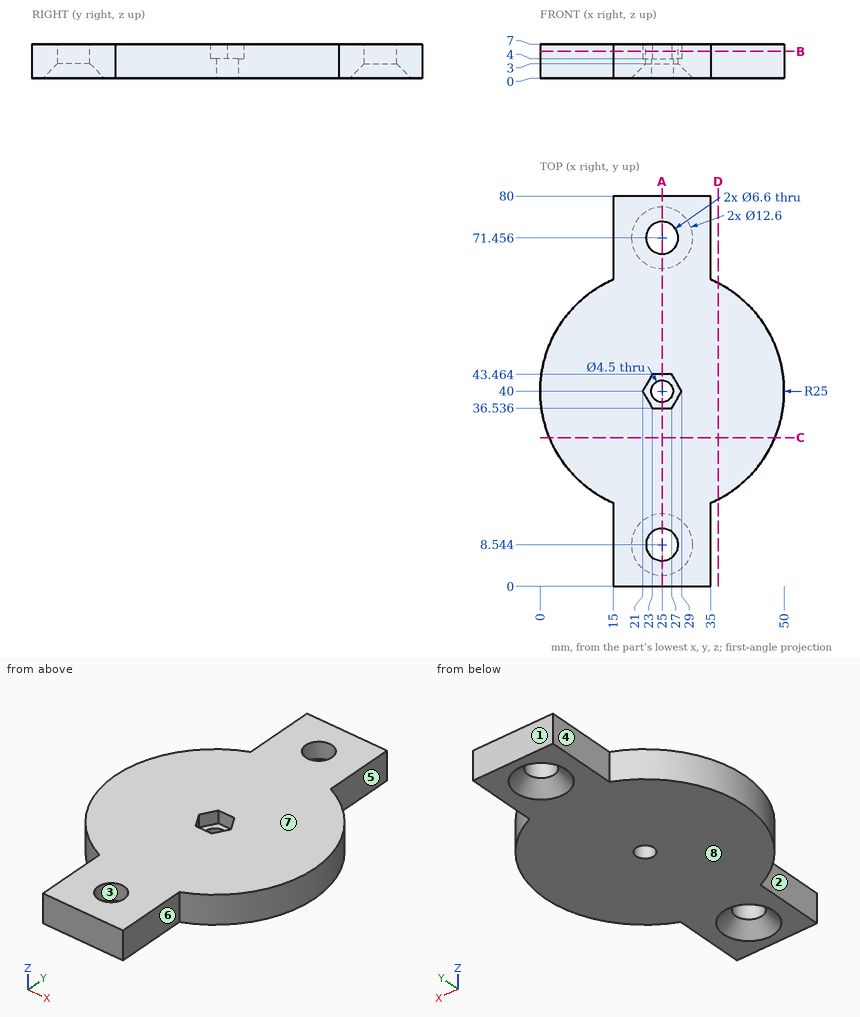
Study the drawing (mm; zero at the part's minimum x, y, z) and answer. A direction names the side the tool comes from. Give positions to 0.01 mm unless a question says otherwise; leave off trailing zeros. Order: outer loops, then holes, each group sorted by start corner. A loop starts at its lowest first (then second) coordinate and runs counter-clockwise, first axis right, second up.
1. The mould has two halves that part along Z. Classify the marked faces 6, 7 and 8: released by +Z, released by -Z, zero draft, split by the parting line, or undercut.
Result sheet:
face 6: zero draft
face 7: released by +Z
face 8: released by -Z
2. For the marked faces 1, 2, 3, 4 and 5, determine the directions among +Z, -Z, +X, -X, +Y, -Y from which every point of the face is accessible in a straight line to the end or side of a thin tool.
Result sheet:
face 1: +Z, -Z, +X, -X, +Y
face 2: +Z, -Z, -X, -Y
face 3: +Z, -Z
face 4: +Z, -Z, -X, +Y
face 5: +Z, -Z, +X, +Y
3. Section A-A, the plane x = 25 is taken. Determine the outline of the cut face in (y, z), and give its area (3 significant figures).
Result sheet:
outline: (0, 0) - (2.24, 0) - (5.24, 3) - (5.24, 7) - (0, 7) - close; (11.84, 3) - (14.84, 0) - (37.75, 0) - (37.75, 4) - (36.54, 4) - (36.54, 7) - (11.84, 7) - close; (42.25, 0) - (65.16, 0) - (68.16, 3) - (68.16, 7) - (43.46, 7) - (43.46, 4) - (42.25, 4) - close; (74.76, 3) - (77.76, 0) - (80, 0) - (80, 7) - (74.76, 7) - close
area: 411 mm2
4. Section C-C, the plane y = 30.5 is taken. Determine the outline of the cut face in (x, z) (1 decimal), and give its area (3 significant figures).
Result sheet:
outline: (1.9, 0) - (48.1, 0) - (48.1, 7) - (1.9, 7) - close
area: 324 mm2
5. Section B-B, the plane z = 5.5 is taken. Determine the outline of the cut face in (x, y).
Result sheet:
outline: (15, 0) - (35, 0) - (35, 17.09) arc R25 ccw to (35, 62.91) - (35, 80) - (15, 80) - (15, 62.91) arc R25 ccw to (15, 17.09) - close; hole (21, 40) - (23, 36.54) - (27, 36.54) - (29, 40) - (27, 43.46) - (23, 43.46) - close; hole circle Ø6.6 at (25, 8.54); hole circle Ø6.6 at (25, 71.46)
6. Each of these flat-tipped pins is pushed along its axis until it touches: P1, Ø3.5, axis at x = 26.5, y = 39.5, coming from the +Z side; P2, Ø10.5, axis at x = 25, y = 71.46, coming from the -Z side (1 decimal); P3, Ø2, axis at y = 47, z = 4, coming from the -X side; P4, Ø2.5, axis at x = 25, y = 40, coming from the +Z side. Where does it stop, or does it pass through?
Result sheet:
P1: stops at z = 4
P2: stops at z = 1
P3: stops at x = 0.73
P4: passes through
7. Section D-D, the plane x = 36.5 is taken. Determine the outline of the cut face in (y, z).
Result sheet:
outline: (17.8, 0) - (62.2, 0) - (62.2, 7) - (17.8, 7) - close
8. Straight lines are drawn through the part: L1, parallel to Y at x = 25, z = 4.65; L2, parallel to Y at x = 22.5, z = 4.75 (1 decimal); L3, parallel to X at y = 17, z = 3.5. For each, find the intervals that lie inside material, in ascending order.
Result sheet:
L1: y = 0 to 5.24, 11.84 to 36.54, 43.46 to 68.16, 74.76 to 80
L2: y = 0 to 6.4, 10.7 to 37.4, 42.6 to 69.3, 73.6 to 80
L3: x = 15 to 35
